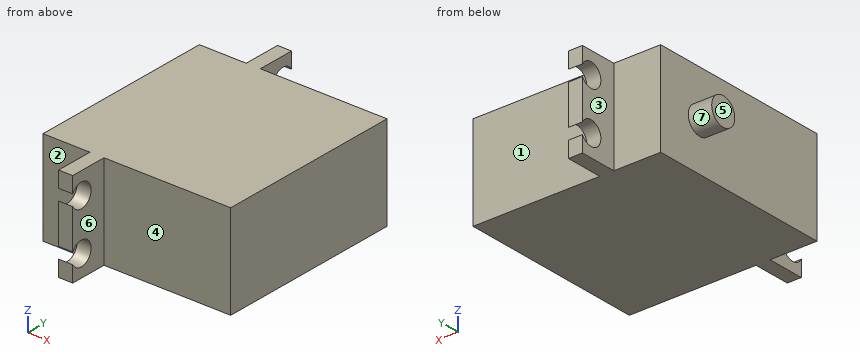
```python
from build123d import *

# Parameters (mm, degrees)
ESQUISSE1_W              = 40
ESQUISSE1_H              = 40
BOSS_EXTRU_1_DEPTH       = 20
ESQUISSE2_W              = 3
ESQUISSE2_H              = 20
BOSS_EXTRU_2_DEPTH       = 8
ESQUISSE3_W              = 3
ESQUISSE3_H              = 20
BOSS_EXTRU_4_DEPTH       = 8
ESQUISSE5_R              = 2.5
ENL_V_MAT_EXTRU_9_DEPTH  = 8
ESQUISSE6_R              = 2.5
ENL_V_MAT_EXTRU_10_DEPTH = 8
ESQUISSE7_R              = 2.95
BOSS_EXTRU_5_DEPTH       = 5


with BuildPart() as part:
    # Esquisse1 → Boss.-Extru.1 (new body)
    with BuildSketch(Plane.XY):
        Rectangle(ESQUISSE1_W, ESQUISSE1_H)
    extrude(amount=BOSS_EXTRU_1_DEPTH)

    # Esquisse2 → Boss.-Extru.2 (add)
    with BuildSketch(Plane(origin=(0, 20, 0), x_dir=(1, 0, 0), z_dir=(0, 1, 0))):
        with Locations((-8.5, -10)):
            Rectangle(ESQUISSE2_W, ESQUISSE2_H)
    extrude(amount=BOSS_EXTRU_2_DEPTH)

    # Esquisse3 → Boss.-Extru.4 (add)
    with BuildSketch(Plane.XZ.offset(20)):
        with Locations((-8.5, 10)):
            Rectangle(ESQUISSE3_W, ESQUISSE3_H)
    extrude(amount=BOSS_EXTRU_4_DEPTH)

    # Esquisse5 → Enlèv. mat.-Extru.9 (cut)
    with BuildSketch(Plane.ZY.offset(10)):
        with Locations((4.6, -25.8)):
            Circle(ESQUISSE5_R)
        with Locations((15.4, -25.8)):
            Circle(ESQUISSE5_R)
    extrude(amount=-ENL_V_MAT_EXTRU_9_DEPTH, mode=Mode.SUBTRACT)

    # Esquisse6 → Enlèv. mat.-Extru.10 (cut)
    with BuildSketch(Plane.ZY.offset(10)):
        with Locations((4.6, 25.8)):
            Circle(ESQUISSE6_R)
        with Locations((15.4, 25.8)):
            Circle(ESQUISSE6_R)
    extrude(amount=-ENL_V_MAT_EXTRU_10_DEPTH, mode=Mode.SUBTRACT)

    # Esquisse7 → Boss.-Extru.5 (add)
    with BuildSketch(Plane.ZY.offset(20)):
        with Locations(Location((10, 10, 0), (0, 0, 180))):
            Circle(ESQUISSE7_R)
    extrude(amount=BOSS_EXTRU_5_DEPTH)


solid = part.part
```
Design review of the part built by this model. Coordinates are the model's own, in mm. Face numbers are marked on the shaded views. A direction names the side the tool comes from. Give positions to 0.01 mm unless a question says otherwise; leave off trailing zeros. Write each loop counter-clockwise with the first axis right and the second up, starting at its lowest first coordinate (ties: lowest second). Pieces come first, ordered by that corner, then holes. Notation, with made-up numbers: (63, -28.5) -> (121, -28.5) arc R22 cw to (121, -3.5) -> close; hole circle Ø2 at (-27.75, 55). An arc over 180 degrees is marked (long way). Answer in a Markdown table with one row per item.
(1) Consider section C-C (x = -8). State the section outline as (y, z) points.
Results:
| item | result |
|---|---|
| outline | (-28, 0) -> (28, 0) -> (28, 3.41) arc R2.5 cw (long way) to (28, 5.79) -> (28, 14.21) arc R2.5 cw (long way) to (28, 16.59) -> (28, 20) -> (-28, 20) -> (-28, 16.59) arc R2.5 cw (long way) to (-28, 14.21) -> (-28, 5.79) arc R2.5 cw (long way) to (-28, 3.41) -> close |
(2) Consider section B-B (z = 15.4). State the section outline as (x, y) points.
Results:
| item | result |
|---|---|
| outline | (-20, -20) -> (-10, -20) -> (-10, -23.3) -> (-7, -23.3) -> (-7, -20) -> (20, -20) -> (20, 20) -> (-7, 20) -> (-7, 23.3) -> (-10, 23.3) -> (-10, 20) -> (-20, 20) -> close |
(3) For the marked faces 1, 2, 3 and 4, list the 3-axis set-ups (+Z, -Z, +X, -X, +Y, -Y) from which the entire face can be reached by the end or side of a thin tool; tool diameter is ignored.
Results:
| item | result |
|---|---|
| face 1 | +Z, -Z, +X, +Y |
| face 2 | +Z, -Z, -X, -Y |
| face 3 | +Z, -Z, -X, +Y |
| face 4 | +Z, -Z, +X, -Y |
(4) Consider section D-D (y = -6.5). State the section outline as (x, z) points, then the cut area to 3 significant figures.
Results:
| item | result |
|---|---|
| outline | (-20, 0) -> (20, 0) -> (20, 20) -> (-20, 20) -> close |
| area | 800 mm2 |
(5) Clearance check with flat-ended pins moving along their axes: pin 1 (4.5 mm diameter, centred on y = 25.8, z = 4.6, fed in from +X); pin 2 (6.5 mm diameter, centred on y = 25.8, z = 15.4, fed in from +X); pin 3 (6 mm diameter, centred on x = 9.5, z = 10.5, fed in from -Y); pin 4 (10 mm diameter, centred on x = 2, z = 7.5, fed in from +Y). State where each tip first meets the part, or that it passes through.
Results:
| item | result |
|---|---|
| pin 1 | through |
| pin 2 | x = -7 |
| pin 3 | y = -20 |
| pin 4 | y = 20 |
(6) To check wall thickness, follow probe 1 along Z at (x, y) = (-7.9, 25.8); probe 2 along X at (y, z) = (-18, 13.75); probe 3 along Z at (x, y) = (-8, 25). State the ranges of each line that lie inside material, in increasing order.
Results:
| item | result |
|---|---|
| probe 1 | 0 to 2.1, 7.1 to 12.9, 17.9 to 20 |
| probe 2 | -20 to 20 |
| probe 3 | 0 to 2.23, 6.97 to 13.03, 17.77 to 20 |
(7) Consider section A-A (y = -25.8). State the section outline as (x, z) points, then the cut area to 3 significant figures.
Results:
| item | result |
|---|---|
| outline | (-10, 0) -> (-7, 0) -> (-7, 2.1) -> (-10, 2.1) -> close; (-10, 7.1) -> (-7, 7.1) -> (-7, 12.9) -> (-10, 12.9) -> close; (-10, 17.9) -> (-7, 17.9) -> (-7, 20) -> (-10, 20) -> close |
| area | 30.0 mm2 |
(8) Mouldability with a two-part tool opening along X and no side actions: class the marked faces 5, 6 and 7 as +X half, -X half, draft (parallel to the pull), parting line (faces both ways), or undercut.
Results:
| item | result |
|---|---|
| face 5 | -X half |
| face 6 | +X half |
| face 7 | draft |
